For this review, take the finished solid that the model builds, in its own axes (mm). A direction names the side the tool comes from. Give positions to 0.01 mm unless a question says otherwise; leave off trailing zeros. Loops run counter-clockwise (first coordinate to the right, second up) from the corner with the lowest first, then second, coordinate; pieces in that order, holes last. Notation, with made-up numbers: (37, -36) - (52, -36) arc R22 cw to (52, -17) - close; hole circle Ø1 at (30, 89.25). An arc over 180 degrees is marked (long way). Put each result on its own line as item: value.
from build123d import *

# Parameters (mm, degrees)
F0_W      = 20.6375
F0_H      = 14.2875
F1_DEPTH  = 38.1
F2_R      = 4
F3_DEPTH  = 19.05
F6_DEPTH  = 22.61794
F7_R      = 1.651
F8_DEPTH  = 6.604
F9_R      = 2.0828
F10_DEPTH = 25.4
F11_R     = 4.064
F12_DEPTH = 25.4
F13_R     = 0.381
F14_R     = 1.9304
F15_DEPTH = 15.3176
F16_R     = 2.54


with BuildPart() as f1:
    # F0 (on Top) → F1 (new body)
    with BuildSketch(Plane.XY):
        with Locations((-2.38125, -0.79375)):
            Rectangle(F0_W, F0_H)
    extrude(amount=F1_DEPTH)

    # F2 (on Top) → F3 (cut)
    with BuildSketch(Plane.XY):
        Circle(F2_R)
    extrude(amount=F3_DEPTH, mode=Mode.SUBTRACT)

    # F5 (on offset) → F6 (cut)
    with BuildSketch(Plane.XZ.offset(0.254)):
        Polygon((-24.257, 41.275), (-24.257, 2.9434311857), (3.8757620392, 31.0761932248), (1.143, 41.275), align=None)
    extrude(amount=-F6_DEPTH, mode=Mode.SUBTRACT)

    # F7 (on face) → F8 (cut, through all)
    with BuildSketch(Plane(origin=(0, 6.35, 0), x_dir=(-1, 0, 0), z_dir=(0, 1, 0))):
        with Locations((-2.7197583304, 31.9964899328)):
            Circle(F7_R)
    extrude(amount=-F8_DEPTH, mode=Mode.SUBTRACT)

    # F9 (on face) → F10 (cut)
    with BuildSketch(Plane(origin=(0, 6.35, 0), x_dir=(-1, 0, 0), z_dir=(0, 1, 0))):
        with Locations((-0.254, 24.4011441045)):
            Circle(F9_R)
        with Locations((8.8952870812, 34.29)):
            Circle(F9_R)
    extrude(amount=-F10_DEPTH, mode=Mode.SUBTRACT)

    # F11 (on face) → F12 (cut)
    with BuildSketch(Plane(origin=(0, -0.254, 0), x_dir=(-1, 0, 0), z_dir=(0, 1, 0))):
        with Locations((-0.254, 24.4011441045)):
            Circle(F11_R)
    extrude(amount=F12_DEPTH, mode=Mode.SUBTRACT)

    # F13
    f13_edges = [f1.edges().sort_by_distance(p)[0] for p in [
        (-3.70727, 3.048, 23.493161),
        (1.161983, 3.048, 28.362414),
        (1.993739, 3.048, 38.1),
    ]]
    fillet(f13_edges, radius=F13_R)

    # F14 (on face) → F15 (cut)
    with BuildSketch(Plane(origin=(-12.7, 0, 0), x_dir=(0, -1, 0), z_dir=(-1, 0, 0))):
        with Locations((0, 9.525)):
            Circle(F14_R)
    extrude(amount=-F15_DEPTH, mode=Mode.SUBTRACT)

    # F16
    f16_edges = [f1.edges().sort_by_distance(p)[0] for p in [
        (-12.7, -4.09575, 38.1),
        (7.9375, -0.79375, 38.1),
    ]]
    fillet(f16_edges, radius=F16_R)


solid = f1.part
1) Insertion check: pin 1 Ø3 at (x, y) = (-1, 4) entering from +Z; pin 2 Ø6.5 at (x, z) = (0.25, 24.4) entering from -Y. Each pin has a flat end and moves straight along its axis. Give the tip position at first contact, or say it passes through.
Geometry check:
pin 1: stops at z = 21.41
pin 2: stops at y = -7.94
2) Take a section at C-C on x = 0.75. State the section outline as (y, z) points.
Geometry check:
outline: (-7.94, 0) - (-3.93, 0) - (-3.93, 19.05) - (3.93, 19.05) - (3.93, 0) - (6.35, 0) - (6.35, 20.37) - (-0.25, 20.37) - (-0.25, 22.38) - (-7.94, 22.38) - close; (-7.94, 26.42) - (-0.25, 26.42) - (-0.25, 38.1) - (-7.94, 38.1) - close
3) Take a section at D-D on z = 34.29. State the section outline as (x, y) points, and give its area (3 significant figures).
Geometry check:
outline: (-12.7, -7.94) - (-10.98, -7.94) - (-10.98, -0.25) - (-12.7, -0.25) - close; (-6.81, -7.94) - (7.94, -7.94) - (7.94, 6.35) - (3.01, 6.35) - (3.01, -0.25) - (-6.81, -0.25) - close
area: 159 mm²
4) Take a section at A-A on y = -1.5. State the section outline as (x, z) points.
Geometry check:
outline: (-12.7, 0) - (-3.71, 0) - (-3.71, 8.31) - (-12.7, 8.31) - close; (-12.7, 10.74) - (-3.71, 10.74) - (-3.71, 19.05) - (3.71, 19.05) - (3.71, 0) - (7.94, 0) - (7.94, 35.56) arc R2.54 ccw to (5.4, 38.1) - (-10.16, 38.1) arc R2.54 ccw to (-12.7, 35.56) - close; hole circle Ø4.17 at (-8.9, 34.29); hole circle Ø4.17 at (0.25, 24.4)
5) Wall thickness on line 1 (X direction, y = -1.25, z = 24.5); line 2 (Y direction, x = 0, z = 11); line 3 (Z direction, x = 0.25, y = -1): over which ranges is each line inside the solid? List them lowest first.
Geometry check:
line 1: x = -12.7 to -1.83, 2.33 to 7.94
line 2: y = -7.94 to -4, 4 to 6.35
line 3: z = 19.05 to 22.32, 26.48 to 38.1
6) For faces 1 (the face through (-8.5, 3, 18.7)), 2 (the face through (0, 0, 19.05)), 3 (the face through (-12.7, -2, 14)), 4 (the face through (2.67, 3, 35.57)), 5 (the face through (0, 6.35, 15)), list the 3-axis set-ups (+Z, -Z, +X, -X, +Y, -Y) from which the entire face can be reached by the end or side of a thin tool; tool diameter is ignored.
Geometry check:
face 1: +Z, -X, +Y
face 2: -Z
face 3: +Z, -Z, -X, +Y, -Y
face 4: -X, +Y
face 5: +Z, -Z, +X, -X, +Y
7) Take a section at B-B on z = 13.5. State the section outline as (x, y) points.
Geometry check:
outline: (-12.7, -7.94) - (7.94, -7.94) - (7.94, 6.35) - (-12.7, 6.35) - close; hole circle Ø8 at (0, 0)
8) Draft analysis for pull direction X (two halves, no side actions). For faces 6 (the face through (7.17, -0.69, 37.38)), 7 (the face through (3.2, 3, 21.6)), 8 (the face through (-8.17, 0.25, 11.44)), state which applies: pulls with the +X half, pulls with the -X half, needs draft (parallel to the pull), parting line crosses it, or undercut.
Geometry check:
face 6: pulls with the +X half
face 7: undercut
face 8: needs draft
